from build123d import *

# Parameters (mm, degrees)
SKETCH2_R          = 3
CUT_EXTRUDE2_DEPTH = 10


with BuildPart() as part:
    # Sketch1 → Revolve1 (revolve)
    with BuildSketch(Plane.XY, mode=Mode.PRIVATE) as revolve1_sk:
        with BuildLine():
            Line((100, 2.844477336), (100, 0))
            add(Edge.make_bspline(
                [(100, 0), (90.312762525, 0), (43.119706996, 15.073582884), (9.43857005, 32.11606328), (3.5, 40.928765801), (3.5, 41.163912301)],
                knots=[0, 0, 0, 0, 0.641468737, 0.741468737, 1, 1, 1, 1], degree=3))
            Line((3.5, 41.163912301), (3.5, 60))
            Line((3.5, 60), (7.057288072, 60))
            Line((7.057288072, 60), (7.057288072, 52.125008745))
            add(Edge.make_bspline(
                [(100, 2.844477336), (58.263448469, 15.906011625), (27.953606397, 25.195125562), (7.057288072, 41.21441144), (7.057288072, 52.125008745)],
                knots=[0, 0, 0, 0, 0.525870122, 1, 1, 1, 1], degree=3))
        make_face()
    revolve(revolve1_sk.sketch.rotate(Axis((0, 82.920033306, 0), (0, -1, 0)), 90), axis=Axis((0, 82.920033306, 0), (0, -1, 0)))

    # Sketch2 → Cut-Extrude2 (cut)
    with BuildSketch(Plane(origin=(0, 0, 0), x_dir=(1, 0, 0), z_dir=(0, 1, 0))):
        with Locations(Location((-50, -50, 0), (0, 0, 90))):
            Circle(SKETCH2_R)
        with Locations(Location((50, -50, 0), (0, 0, 90))):
            Circle(SKETCH2_R)
        with Locations(Location((50, 50, 0), (0, 0, 90))):
            Circle(SKETCH2_R)
        with Locations(Location((-50, 50, 0), (0, 0, 90))):
            Circle(SKETCH2_R)
    extrude(amount=CUT_EXTRUDE2_DEPTH, mode=Mode.SUBTRACT)


solid = part.part
Can you work these out from the model? Positions are in its coordinate system, mm. A direction names the side the tool comes from. Coordinates: 2 decimals unless noted, no trailing zeros.
Q1. Which directions (+Z, -Z, +X, -X, +Y, -Y) give clear straight access to the entire face, cutting with the end or side of a thin tool? Please do faces 4 (the face through (-30.04, 1.4, 95.38)), 5 (the face through (52.662, 8.475, -51.384)).
Results found:
face 4: +Y, -Y
face 5: -Y
Q2. If we mould it in two halves opening along Z, with no side actions, what happens to faces 1 (the face through (3, 60, -3)), 2 (the face through (-2.12, 56.01, 6.73)), 3 (the face through (-52.03, 8.47, 52.21))? For each: +Z half, -Z half, draft (parallel to the pull), parting line (faces both ways), or undercut.
Results found:
face 1: draft
face 2: parting line
face 3: undercut
Q3. For P1, Ø9.5, axis at x = 50, z = -50, coming from the +Y side; P2, Ø1.8, axis at x = 50.5, z = 48.5, coming from the -Y side; P3, Ø1.5, axis at y = 48, z = 0, coming from the -X side; P4, Ø5.5, axis at x = 0, z = 0, coming from the -Y side, each with a flat end and sliding along its axis, tell me the tip position at first contact or that it passes through.
Results found:
P1: stops at y = 13.57
P2: stops at y = 10
P3: stops at x = -7.75
P4: passes through
Q4. Please list where these lines run through material, in increasing order: L1, parallel to X at y = 45, z = 0; L2, parallel to Z at x = 10, y = 31; L3, parallel to Y at x = 43, z = -71.
Results found:
L1: x = -8.58 to -3.5, 3.5 to 8.58
L2: z = -20.39 to -8.77, 8.77 to 20.39
L3: y = 3.43 to 8.17
